from build123d import *

# Parameters (mm, degrees)
F0_R     = 44
F0_R_2   = 8.1
F1_DEPTH = 15
F2_DEPTH = 50
F3_R     = 5


with BuildPart() as f1:
    # F0 (on Top) → F1 (new body)
    with BuildSketch(Plane.XY):
        Circle(F0_R)
        with BuildLine():
            ThreePointArc((31.2499935607, 0.017853412), (28.0020236485, -5.6101391527), (21.5040550044, -5.6136546355))
            Line((21.5040550044, -5.6136546355), (15.636396845, -15.7936884136))
            ThreePointArc((15.636396845, -15.7936884136), (18.0184508533, -18.1731663733), (18.8904582887, -21.4251964611))
            ThreePointArc((18.8904582887, -21.4251964611), (12.3928026762, -27.9251960383), (5.8904599798, -21.429885236))
            Line((5.8904599798, -21.429885236), (-5.8595369632, -21.4383610982))
            ThreePointArc((-5.8595369632, -21.4383610982), (-5.8595356948, -21.4407054855), (-5.8595352721, -21.4430498731))
            ThreePointArc((-5.8595352721, -21.4430498731), (-15.6075047615, -27.0733868253), (-15.6135950246, -15.8162306005))
            Line((-15.6135950246, -15.8162306005), (-21.4959338081, -5.6446726846))
            ThreePointArc((-21.4959338081, -5.6446726846), (-31.2499918696, -0.0225421868), (-21.5040550044, 5.6136546355))
            Line((-21.5040550044, 5.6136546355), (-15.636396845, 15.7936884136))
            ThreePointArc((-15.636396845, 15.7936884136), (-15.6445180412, 27.0520157337), (-5.8904599798, 21.429885236))
            Line((-5.8904599798, 21.429885236), (5.8595369632, 21.4383610982))
            ThreePointArc((5.8595369632, 21.4383610982), (12.3571908845, 27.9430494503), (18.8595352721, 21.4430498731))
            ThreePointArc((18.8595352721, 21.4430498731), (17.9898722243, 18.1950803837), (15.6135950246, 15.8162306005))
            Line((15.6135950246, 15.8162306005), (21.4959338081, 5.6446726846))
            ThreePointArc((21.4959338081, 5.6446726846), (27.9979630501, 5.6481903642), (31.2499935607, 0.017853412))
        make_face(mode=Mode.SUBTRACT)
        with BuildLine():
            Line((15.636396845, -15.7936884136), (21.5040550044, -5.6136546355))
            ThreePointArc((21.5040550044, -5.6136546355), (18.2499952518, 0.0131646371), (21.4959338081, 5.6446726846))
            Line((21.4959338081, 5.6446726846), (15.6135950246, 15.8162306005))
            ThreePointArc((15.6135950246, 15.8162306005), (9.1135967158, 15.8115418256), (5.8595369632, 21.4383610982))
            Line((5.8595369632, 21.4383610982), (-5.8904599798, 21.429885236))
            ThreePointArc((-5.8904599798, 21.429885236), (-5.8904587114, 21.4275408487), (-5.8904582887, 21.4251964611))
            ThreePointArc((-5.8904582887, 21.4251964611), (-9.1384282009, 15.7972038964), (-15.636396845, 15.7936884136))
            Line((-15.636396845, 15.7936884136), (-21.5040550044, 5.6136546355))
            ThreePointArc((-21.5040550044, 5.6136546355), (-19.1220009961, 3.2341766758), (-18.2499935607, -0.017853412))
            ThreePointArc((-18.2499935607, -0.017853412), (-19.1196566085, -3.2658229014), (-21.4959338081, -5.6446726846))
            Line((-21.4959338081, -5.6446726846), (-15.6135950246, -15.8162306005))
            ThreePointArc((-15.6135950246, -15.8162306005), (-9.1135967158, -15.8115418256), (-5.8595369632, -21.4383610982))
            Line((-5.8595369632, -21.4383610982), (5.8904599798, -21.429885236))
            ThreePointArc((5.8904599798, -21.429885236), (9.1363985361, -15.7983771885), (15.636396845, -15.7936884136))
        make_face()
        Circle(F0_R_2, mode=Mode.SUBTRACT)
    extrude(amount=F1_DEPTH)

    # F0 (on Top) → F2 (join)
    with BuildSketch(Plane.XY):
        Circle(F0_R)
        with BuildLine():
            ThreePointArc((31.2499935607, 0.017853412), (28.0020236485, -5.6101391527), (21.5040550044, -5.6136546355))
            Line((21.5040550044, -5.6136546355), (15.636396845, -15.7936884136))
            ThreePointArc((15.636396845, -15.7936884136), (18.0184508533, -18.1731663733), (18.8904582887, -21.4251964611))
            ThreePointArc((18.8904582887, -21.4251964611), (12.3928026762, -27.9251960383), (5.8904599798, -21.429885236))
            Line((5.8904599798, -21.429885236), (-5.8595369632, -21.4383610982))
            ThreePointArc((-5.8595369632, -21.4383610982), (-5.8595356948, -21.4407054855), (-5.8595352721, -21.4430498731))
            ThreePointArc((-5.8595352721, -21.4430498731), (-15.6075047615, -27.0733868253), (-15.6135950246, -15.8162306005))
            Line((-15.6135950246, -15.8162306005), (-21.4959338081, -5.6446726846))
            ThreePointArc((-21.4959338081, -5.6446726846), (-31.2499918696, -0.0225421868), (-21.5040550044, 5.6136546355))
            Line((-21.5040550044, 5.6136546355), (-15.636396845, 15.7936884136))
            ThreePointArc((-15.636396845, 15.7936884136), (-15.6445180412, 27.0520157337), (-5.8904599798, 21.429885236))
            Line((-5.8904599798, 21.429885236), (5.8595369632, 21.4383610982))
            ThreePointArc((5.8595369632, 21.4383610982), (12.3571908845, 27.9430494503), (18.8595352721, 21.4430498731))
            ThreePointArc((18.8595352721, 21.4430498731), (17.9898722243, 18.1950803837), (15.6135950246, 15.8162306005))
            Line((15.6135950246, 15.8162306005), (21.4959338081, 5.6446726846))
            ThreePointArc((21.4959338081, 5.6446726846), (27.9979630501, 5.6481903642), (31.2499935607, 0.017853412))
        make_face(mode=Mode.SUBTRACT)
        with BuildLine():
            Line((15.636396845, -15.7936884136), (21.5040550044, -5.6136546355))
            ThreePointArc((21.5040550044, -5.6136546355), (18.2499952518, 0.0131646371), (21.4959338081, 5.6446726846))
            Line((21.4959338081, 5.6446726846), (15.6135950246, 15.8162306005))
            ThreePointArc((15.6135950246, 15.8162306005), (9.1135967158, 15.8115418256), (5.8595369632, 21.4383610982))
            Line((5.8595369632, 21.4383610982), (-5.8904599798, 21.429885236))
            ThreePointArc((-5.8904599798, 21.429885236), (-5.8904587114, 21.4275408487), (-5.8904582887, 21.4251964611))
            ThreePointArc((-5.8904582887, 21.4251964611), (-9.1384282009, 15.7972038964), (-15.636396845, 15.7936884136))
            Line((-15.636396845, 15.7936884136), (-21.5040550044, 5.6136546355))
            ThreePointArc((-21.5040550044, 5.6136546355), (-19.1220009961, 3.2341766758), (-18.2499935607, -0.017853412))
            ThreePointArc((-18.2499935607, -0.017853412), (-19.1196566085, -3.2658229014), (-21.4959338081, -5.6446726846))
            Line((-21.4959338081, -5.6446726846), (-15.6135950246, -15.8162306005))
            ThreePointArc((-15.6135950246, -15.8162306005), (-9.1135967158, -15.8115418256), (-5.8595369632, -21.4383610982))
            Line((-5.8595369632, -21.4383610982), (5.8904599798, -21.429885236))
            ThreePointArc((5.8904599798, -21.429885236), (9.1363985361, -15.7983771885), (15.636396845, -15.7936884136))
        make_face()
        Circle(F0_R_2, mode=Mode.SUBTRACT)
        Circle(F0_R_2)
        with BuildLine():
            ThreePointArc((-5.8595352721, -21.4430498731), (-5.8595356948, -21.4407054855), (-5.8595369632, -21.4383610982))
            Line((-5.8595369632, -21.4383610982), (-12.3595352721, -21.4430498731))
            Line((-12.3595352721, -21.4430498731), (-15.6135950246, -15.8162306005))
            ThreePointArc((-15.6135950246, -15.8162306005), (-15.6075047615, -27.0733868253), (-5.8595352721, -21.4430498731))
        make_face()
        with BuildLine():
            ThreePointArc((-21.5040550044, 5.6136546355), (-31.2499918696, -0.0225421868), (-21.4959338081, -5.6446726846))
            Line((-21.4959338081, -5.6446726846), (-24.7499935607, -0.017853412))
            Line((-24.7499935607, -0.017853412), (-21.5040550044, 5.6136546355))
        make_face()
        with BuildLine():
            ThreePointArc((18.8904582887, -21.4251964611), (18.0184508533, -18.1731663733), (15.636396845, -15.7936884136))
            Line((15.636396845, -15.7936884136), (12.3904582887, -21.4251964611))
            Line((12.3904582887, -21.4251964611), (5.8904599798, -21.429885236))
            ThreePointArc((5.8904599798, -21.429885236), (12.3928026762, -27.9251960383), (18.8904582887, -21.4251964611))
        make_face()
        with BuildLine():
            Line((21.4959338081, 5.6446726846), (24.7499935607, 0.017853412))
            Line((24.7499935607, 0.017853412), (21.5040550044, -5.6136546355))
            ThreePointArc((21.5040550044, -5.6136546355), (28.0020236485, -5.6101391527), (31.2499935607, 0.017853412))
            ThreePointArc((31.2499935607, 0.017853412), (27.9979630501, 5.6481903642), (21.4959338081, 5.6446726846))
        make_face()
        with BuildLine():
            Line((12.3595352721, 21.4430498731), (15.6135950246, 15.8162306005))
            ThreePointArc((15.6135950246, 15.8162306005), (17.9898722243, 18.1950803837), (18.8595352721, 21.4430498731))
            ThreePointArc((18.8595352721, 21.4430498731), (12.3571908845, 27.9430494503), (5.8595369632, 21.4383610982))
            Line((5.8595369632, 21.4383610982), (12.3595352721, 21.4430498731))
        make_face()
        with BuildLine():
            Line((-12.3904582887, 21.4251964611), (-5.8904599798, 21.429885236))
            ThreePointArc((-5.8904599798, 21.429885236), (-15.6445180412, 27.0520157337), (-15.636396845, 15.7936884136))
            Line((-15.636396845, 15.7936884136), (-12.3904582887, 21.4251964611))
        make_face()
        with BuildLine():
            Line((-12.3595352721, -21.4430498731), (-5.8595369632, -21.4383610982))
            ThreePointArc((-5.8595369632, -21.4383610982), (-9.1135967158, -15.8115418256), (-15.6135950246, -15.8162306005))
            Line((-15.6135950246, -15.8162306005), (-12.3595352721, -21.4430498731))
        make_face()
        with BuildLine():
            Line((-24.7499935607, -0.017853412), (-21.4959338081, -5.6446726846))
            ThreePointArc((-21.4959338081, -5.6446726846), (-19.1196566085, -3.2658229014), (-18.2499935607, -0.017853412))
            ThreePointArc((-18.2499935607, -0.017853412), (-19.1220009961, 3.2341766758), (-21.5040550044, 5.6136546355))
            Line((-21.5040550044, 5.6136546355), (-24.7499935607, -0.017853412))
        make_face()
        with BuildLine():
            Line((12.3904582887, -21.4251964611), (15.636396845, -15.7936884136))
            ThreePointArc((15.636396845, -15.7936884136), (9.1363985361, -15.7983771885), (5.8904599798, -21.429885236))
            Line((5.8904599798, -21.429885236), (12.3904582887, -21.4251964611))
        make_face()
        with BuildLine():
            Line((21.5040550044, -5.6136546355), (24.7499935607, 0.017853412))
            Line((24.7499935607, 0.017853412), (21.4959338081, 5.6446726846))
            ThreePointArc((21.4959338081, 5.6446726846), (18.2499952518, 0.0131646371), (21.5040550044, -5.6136546355))
        make_face()
        with BuildLine():
            ThreePointArc((-5.8904582887, 21.4251964611), (-5.8904587114, 21.4275408487), (-5.8904599798, 21.429885236))
            Line((-5.8904599798, 21.429885236), (-12.3904582887, 21.4251964611))
            Line((-12.3904582887, 21.4251964611), (-15.636396845, 15.7936884136))
            ThreePointArc((-15.636396845, 15.7936884136), (-9.1384282009, 15.7972038964), (-5.8904582887, 21.4251964611))
        make_face()
        with BuildLine():
            ThreePointArc((5.8595369632, 21.4383610982), (9.1135967158, 15.8115418256), (15.6135950246, 15.8162306005))
            Line((15.6135950246, 15.8162306005), (12.3595352721, 21.4430498731))
            Line((12.3595352721, 21.4430498731), (5.8595369632, 21.4383610982))
        make_face()
    extrude(amount=-F2_DEPTH)

    # F3
    f3_edges = [f1.edges().sort_by_distance(p)[0] for p in [
        (-44, 0, 15),
        (-44, 0, -50),
    ]]
    fillet(f3_edges, radius=F3_R)


solid = f1.part
Input: part model. Units: mm. Frame: model coordinates. A direction names the side the tool comes from. Round coordinates to 2 decimals unless told otherwise and drop trailing zeros. Loops run counter-clockwise (first coordinate to the right, second up) from the corner with the lowest first, then second, coordinate; pieces in that order, holes last. Notation, with made-up numbers: M 82.5,66 L 122.5,66 A21 ccw 122.5,74 Z; hole C 81.25,-37 d4. An arc over 180 degrees is marked long. Answer as CSV lines item,"result". Start each with the question number.
(1) Draft query along Y for faces 1 (the flat face through (-12, 22, 0)), 2 (the flat face through (-1, 1, -50)), 3 (the cylindrical face through (-9.538, -42.954, -17.115)). Return one class per face: released by +Y, released by -Y, zero draft, split by the parting line, or undercut.
(2) First-contact query: pin 1 (5 mm diameter, centred on x = -3.5, y = -2.5, fed in from +Z); pin 2 (1 mm diameter, centred on y = 1.5, z = -12.5, fed in from +X); pin 3 (1.5 mm diameter, centred on x = 25.5, z = -21, fed in from +Y). Flat tips, straight axial feed; report the tip coordinate or a pass-through.
(3) Section B-B, the plane x = 0. Output: boundary loops of the cut face in (y, z), plus the area to 3 significant figures.
(4) Section C-C, the plane z = -26.5. Output: boundary loops of the cut face in (x, y).
(5) Section A-A, the plane z = 6. State how many separate pieces and enclosed holes the cut face has, plus the area to 3 significant figures.
(6) Reachability of faces 4 (the flat face through (-1, 9, 15)), 5 (the flat face through (25, 0, 0)) from +Z, -Z, +X, -X, +Y, -Y: full face, straight path, thin tool, end or side. Return the list, or none.
(7) Line query: line 1 (X direction, y = -15.5, z = 3.5); line 2 (X direction, y = -18, z = 12); line 3 (Y direction, x = 0, z = 5.25). Output: solid intervals per line, ascending. Write a range as [from, to].
Values found:
1,face 1,"undercut"
1,face 2,"zero draft"
1,face 3,"split by the parting line"
2,pin 1,"stops at z = 0"
2,pin 2,"stops at x = 43.99"
2,pin 3,"stops at y = 36.38"
3,outline,"M -44,-45 A5 ccw -39,-50 L 39,-50 A5 ccw 44,-45 L 44,10 A5 ccw 39,15 L 8.1,15 L 8.1,0 L -8.1,0 L -8.1,15 L -39,15 A5 ccw -44,10 Z"
3,area,"5,460 mm²"
4,outline,"C 0,0 d88"
5,separate pieces,"1"
5,enclosed holes,"7"
5,area,"5,080 mm²"
6,face 4,"+Z, +X, -X, +Y, -Y"
6,face 5,"+Z"
7,line 1,"x = [-41.18, -14.99], [-9.73, 9.72], [15.06, 41.18]"
7,line 2,"x = [-39.69, -17.87], [-6.85, 6.87], [17.91, 39.69]"
7,line 3,"y = [-44, -8.1], [8.1, 44]"
